Input: part model. Units: mm. Frame: model coordinates. Round coordinates to 2 decimals unless told otherwise and drop trailing zeros. Loops run counter-clockwise (first coordinate to the right, second up) from the corner with the lowest first, then second, coordinate; pieces in that order, holes last. Notation, with made-up numbers: M -31.75,-33.5 L -0.75,-33.5 A18 cw -0.75,-19.5 Z; hole C -3.75,14.25 d8. An arc over 180 degrees is marked long. Put each result on its own line as item: value. Start each with the question number.
1) Section B-B on z = -24.5. Output: boundary loops of the cut face in (x, y), plus the area to 3 significant figures.
2) Section A-A on z = 14.94. Output: boundary loops of the cut face in (x, y).
3) Line query: probe 1 along X at (y, z) = (0.5, 14.94); probe 2 along X at (y, z) = (0.6, -19); probe 3 along X at (y, z) = (0.9, -23). Output: solid intervals per line, ascending.
4) Section D-D on y = 0.65. State how many separate pieces and enclosed holes the cut face has, plus the area to 3 significant figures.
5) Section C-C on x = 5. Output: boundary loops of the cut face in (y, z), plus the area to 3 significant figures.
from build123d import *

# Parameters (mm, degrees)
ESBO_O1_W                = 115.09677689
ESBO_O1_H                = 63
RESSALTO_EXTRUS_O1_DEPTH = 2
ESBO_O2_R                = 1.55
CORTE_EXTRUS_O1_DEPTH    = 66.635866816
ESBO_O3_W                = 18
ESBO_O3_H                = 6
CORTE_EXTRUS_O2_DEPTH    = 66.635866816
FILETE1_R                = 3
ESBO_O8_R                = 1.2
CORTE_EXTRUS_O4_DEPTH    = 66.635866816
ESBO_O9_R                = 1.5
CORTE_EXTRUS_O5_DEPTH    = 66.635866816


with BuildPart() as part:
    # Esboço1 → Ressalto-extrusão1 (new body)
    with BuildSketch(Plane(origin=(0, 0, 0), x_dir=(1, 0, 0), z_dir=(0, 1, 0))):
        Rectangle(ESBO_O1_W, ESBO_O1_H)
    extrude(amount=RESSALTO_EXTRUS_O1_DEPTH)

    # Esboço2 → Corte-extrusão1 (cut, through all)
    with BuildSketch(Plane(origin=(0, 2, 0), x_dir=(1, 0, 0), z_dir=(0, 1, 0))):
        with Locations(Location((-46.153556516, -14.945, 0), (0, 0, 270))):
            Circle(ESBO_O2_R)
        with Locations(Location((-22.093556516, -14.94, 0), (0, 0, 270))):
            Circle(ESBO_O2_R)
        with Locations(Location((22.093556516, -14.94, 0), (0, 0, 90))):
            Circle(ESBO_O2_R)
        with Locations(Location((46.153556516, -14.945, 0), (0, 0, 90))):
            Circle(ESBO_O2_R)
        with Locations(Location((46.153556516, 14.945, 0), (0, 0, 270))):
            Circle(ESBO_O2_R)
        with Locations(Location((22.093556516, 14.94, 0), (0, 0, 270))):
            Circle(ESBO_O2_R)
        with Locations(Location((-22.093556516, 14.94, 0), (0, 0, 90))):
            Circle(ESBO_O2_R)
        with Locations(Location((-46.153556516, 14.945, 0), (0, 0, 90))):
            Circle(ESBO_O2_R)
    extrude(amount=-CORTE_EXTRUS_O1_DEPTH, mode=Mode.SUBTRACT)

    # Esboço3 → Corte-extrusão2 (cut, through all)
    with BuildSketch(Plane.XZ):
        with Locations((0, 25.5)):
            Rectangle(ESBO_O3_W, ESBO_O3_H)
        with Locations((0, -25.5)):
            Rectangle(ESBO_O3_W, ESBO_O3_H)
    extrude(amount=-CORTE_EXTRUS_O2_DEPTH, mode=Mode.SUBTRACT)

    # Filete1
    filete1_edges = [part.edges().sort_by_distance(p)[0] for p in [
        (-57.548388445, 1, -31.5),
        (57.548388445, 1, -31.5),
        (57.548388445, 1, 31.5),
        (-57.548388445, 1, 31.5),
    ]]
    fillet(filete1_edges, radius=FILETE1_R)

    # Esboço8 → Corte-extrusão4 (cut, through all)
    with BuildSketch(Plane(origin=(0, 2, 0), x_dir=(1, 0, 0), z_dir=(0, 1, 0))):
        with Locations(Location((-12.498388445, 28.5, 0), (0, 0, 270))):
            Circle(ESBO_O8_R)
        with Locations(Location((12.498388445, 28.5, 0), (0, 0, 90))):
            Circle(ESBO_O8_R)
        with Locations(Location((12.498388445, -28.5, 0), (0, 0, 270))):
            Circle(ESBO_O8_R)
        with Locations(Location((-12.498388445, -28.5, 0), (0, 0, 90))):
            Circle(ESBO_O8_R)
        with Locations(Location((-8.998388445, -19, 0), (0, 0, 270))):
            Circle(ESBO_O8_R)
        with Locations(Location((8.998388445, -19, 0), (0, 0, 90))):
            Circle(ESBO_O8_R)
        with Locations(Location((8.998388445, 19, 0), (0, 0, 270))):
            Circle(ESBO_O8_R)
        with Locations(Location((-8.998388445, 19, 0), (0, 0, 90))):
            Circle(ESBO_O8_R)
    extrude(amount=-CORTE_EXTRUS_O4_DEPTH, mode=Mode.SUBTRACT)

    # Esboço9 → Corte-extrusão5 (cut, through all)
    with BuildSketch(Plane(origin=(0, 2, 0), x_dir=(1, 0, 0), z_dir=(0, 1, 0))):
        with Locations(Location((-46, 27.5, 0), (0, 0, 270))):
            Circle(ESBO_O9_R)
        with Locations(Location((46, 27.5, 0), (0, 0, 90))):
            Circle(ESBO_O9_R)
        with Locations(Location((46, -27.5, 0), (0, 0, 270))):
            Circle(ESBO_O9_R)
        with Locations(Location((-46, -27.5, 0), (0, 0, 90))):
            Circle(ESBO_O9_R)
    extrude(amount=-CORTE_EXTRUS_O5_DEPTH, mode=Mode.SUBTRACT)


solid = part.part
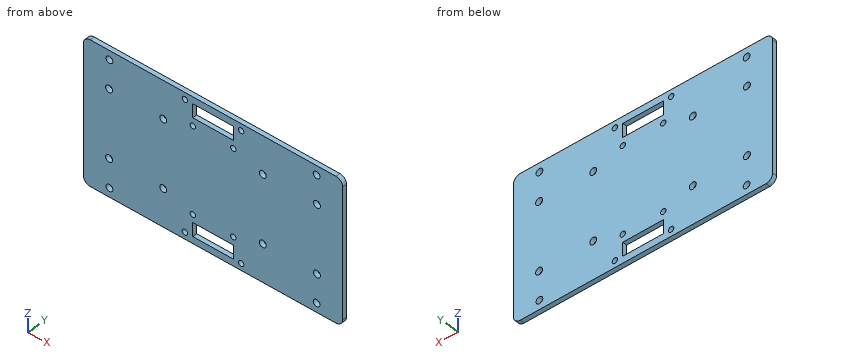
Geometry results:
1. outline: M -57.55,0 L -9,0 L -9,2 L -57.55,2 Z; M 9,0 L 57.55,0 L 57.55,2 L 9,2 Z
1. area: 194 mm²
2. outline: M -57.55,0 L -47.7,0 L -47.7,2 L -57.55,2 Z; M -44.6,0 L -23.64,0 L -23.64,2 L -44.6,2 Z; M -20.54,0 L 20.54,0 L 20.54,2 L -20.54,2 Z; M 23.64,0 L 44.6,0 L 44.6,2 L 23.64,2 Z; M 47.7,0 L 57.55,0 L 57.55,2 L 47.7,2 Z
3. probe 1: x = -57.55 to -47.7, -44.6 to -23.64, -20.54 to 20.54, 23.64 to 44.6, 47.7 to 57.55
3. probe 2: x = -57.55 to -10.2, -7.8 to 7.8, 10.2 to 57.55
3. probe 3: x = -57.55 to -9, 9 to 57.55
4. separate pieces: 1
4. enclosed holes: 22
4. area: 6,900 mm²
5. outline: M 0,-31.5 L 2,-31.5 L 2,-28.5 L 0,-28.5 Z; M 0,-22.5 L 2,-22.5 L 2,22.5 L 0,22.5 Z; M 0,28.5 L 2,28.5 L 2,31.5 L 0,31.5 Z
5. area: 102 mm²
